from build123d import *
from OCP.BRepFilletAPI import BRepFilletAPI_MakeFillet

# Parameters (mm, degrees)
SKETCH1_W           = 59.944
SKETCH1_H           = 34.798
BOSS_EXTRUDE1_DEPTH = 10.16
FILLET1_R           = 2.032
SKETCH2_R           = 7.62
BOSS_EXTRUDE2_DEPTH = 3.81
FILLET2_R1          = 0.254
FILLET2_R2          = 0.762
SKETCH3_R           = 2.413
BOSS_EXTRUDE3_DEPTH = 17.78
SKETCH4_W           = 9.652
SKETCH4_H           = 8.001
BOSS_EXTRUDE4_DEPTH = 13.335
SKETCH5_W           = 9.652
SKETCH5_H           = 8.001
BOSS_EXTRUDE5_DEPTH = 15.748
BOSS_EXTRUDE5_TAPER = 3.5
SKETCH6_R           = 1.905
BOSS_EXTRUDE6_DEPTH = 15.748
SKETCH7_W           = 35.955959778
SKETCH7_H           = 18.169743528
CUT_EXTRUDE1_DEPTH  = 0.00254


with BuildPart() as part:
    # Sketch1 → Boss-Extrude1 (new, symmetric)
    with BuildSketch(Plane(origin=(0, 0, 0), x_dir=(1, 0, 0), z_dir=(0, 1, 0))):
        Rectangle(SKETCH1_W, SKETCH1_H)
    extrude(amount=BOSS_EXTRUDE1_DEPTH, both=True)

    # Fillet1
    fillet1_edges = [part.edges().sort_by_distance(p)[0] for p in [
        (-29.972, 10.16, 0),
        (0, 10.16, 17.399),
        (29.972, 10.16, 0),
        (0, -10.16, 17.399),
        (-29.972, -10.16, 0),
        (0, -10.16, -17.399),
        (29.972, -10.16, 0),
        (0, 10.16, -17.399),
        (29.972, 0, 17.399),
        (-29.972, 0, 17.399),
        (-29.972, 0, -17.399),
        (29.972, 0, -17.399),
    ]]
    fillet(fillet1_edges, radius=FILLET1_R)

    # Sketch2 → Boss-Extrude2 (add)
    with BuildSketch(Plane.ZY.offset(29.972)):
        with Locations(Location((0, 0, 0), (0, 0, 180))):
            Circle(SKETCH2_R)
    extrude(amount=BOSS_EXTRUDE2_DEPTH)

    # Fillet2: one fillet with a radius per group of edges: ONE call of the kernel's fillet builder (fillet() takes one radius for all edges)
    fillet2_edges_1 = [part.edges().sort_by_distance(p)[0] for p in [
        (-33.782, 0, 7.62),
    ]]
    fillet2_edges_2 = [part.edges().sort_by_distance(p)[0] for p in [
        (-29.972, 0, 7.62),
    ]]
    fillet2 = BRepFilletAPI_MakeFillet(part.part.solid().wrapped)
    for e in fillet2_edges_1:
        fillet2.Add(FILLET2_R1, e.wrapped)
    for e in fillet2_edges_2:
        fillet2.Add(FILLET2_R2, e.wrapped)
    add(Compound.cast(fillet2.Shape()), mode=Mode.REPLACE)

    # Sketch3 → Boss-Extrude3 (add)
    with BuildSketch(Plane.ZY.offset(33.782)):
        with Locations((1.819787166, 0)):
            Circle(SKETCH3_R)
    extrude(amount=BOSS_EXTRUDE3_DEPTH)

    # Sketch4 → Boss-Extrude4 (add)
    with BuildSketch(Plane(origin=(29.972, 0, 0), x_dir=(0, 0, -1), z_dir=(1, 0, 0))):
        Rectangle(SKETCH4_W, SKETCH4_H)
    extrude(amount=BOSS_EXTRUDE4_DEPTH)

    # Sketch5 → Boss-Extrude5 (add)
    with BuildSketch(Plane(origin=(43.307, 0, 0), x_dir=(0, 0, -1), z_dir=(1, 0, 0))):
        Rectangle(SKETCH5_W, SKETCH5_H)
    extrude(amount=BOSS_EXTRUDE5_DEPTH, taper=BOSS_EXTRUDE5_TAPER)

    # Sketch6 → Boss-Extrude6 (add)
    with BuildSketch(Plane(origin=(59.055, 0, 0), x_dir=(0, 0, -1), z_dir=(1, 0, 0))):
        Circle(SKETCH6_R)
    extrude(amount=BOSS_EXTRUDE6_DEPTH)

    # Sketch7 → Cut-Extrude1 (cut)
    with BuildSketch(Plane(origin=(0, 10.16, 0), x_dir=(1, 0, 0), z_dir=(0, 1, 0))):
        Rectangle(SKETCH7_W, SKETCH7_H)
    extrude(amount=-CUT_EXTRUDE1_DEPTH, mode=Mode.SUBTRACT)


solid = part.part
Geometry: final body of the model. Coordinates: model frame, mm. A direction names the side the tool comes from. Give positions to 0.01 mm unless a question says otherwise; leave off trailing zeros. Write each loop counter-clockwise with the first axis right and the second up, starting at its lowest first coordinate (ties: lowest second). Pieces come first, ordered by that corner, then holes. Notation, with made-up numbers: (62, -15) - (120, -15) arc R22 cw to (120, -8) - close; hole circle Ø3 at (45.25, 8). An arc over 180 degrees is marked (long way). Return JSON: item names as keys, results as strings. Group by question number.
1) Set-up query: faces 1 (the flat face through (37, 4, 0)), 2 (the flat face through (0, 10.157, 0)), 3 (the cylindrical face through (-32.102, -7.555, 0.992)), 4 (the flat face through (37, 0, 4.826)), 5 (the flat face through (0, 0, 17.399)). Return all of +Z, -Z, +X, -X, +Y, -Y with unobstructed straight access to the full face (end or side cutting, diameter ignored); none if empty.
2) Line query: line 1 (X direction, y = -5.5, z = 14); line 2 (X direction, y = -4.25, z = 3.5); line 3 (Y direction, x = -0.5, z = -7.5). Output: solid intervals per line, ascending.
3) Section A-A on z = -13.5. Return the cut outline in (x, y), plus the area to 3 significant figures.
4) First-contact query: P1, Ø6, axis at y = -4.5, z = -10.5, coming from the +X side; P2, Ø10.5, axis at y = -3.5, z = -6, coming from the -X side; P3, Ø6.5, axis at x = 35, y = 2, coming from the +Z side. Flat tips, straight axial feed; report the tip coordinate or a pass-through.
Filled in:
{
 "1": {"face 1": "+Z, -Z, +X, +Y", "face 2": "+Z, -Z, +X, -X, +Y", "face 3": "-X", "face 4": "+Z, +X, +Y, -Y", "face 5": "+Z, +X, -X, +Y, -Y"},
 "2": {"line 1": "x = -29.97 to 29.97", "line 2": "x = -33.78 to 29.97", "line 3": "y = -10.16 to 10.16"},
 "3": {"outline": "(-29.97, -8.13) arc R2.03 ccw to (-27.94, -10.16) - (27.94, -10.16) arc R2.03 ccw to (29.97, -8.13) - (29.97, 8.13) arc R2.03 ccw to (27.94, 10.16) - (-27.94, 10.16) arc R2.03 ccw to (-29.97, 8.13) - close", "area": "1,210 mm^2"},
 "4": {"P1": "stops at x = 29.97", "P2": "stops at x = -33.78", "P3": "stops at z = 4.83"}
}
